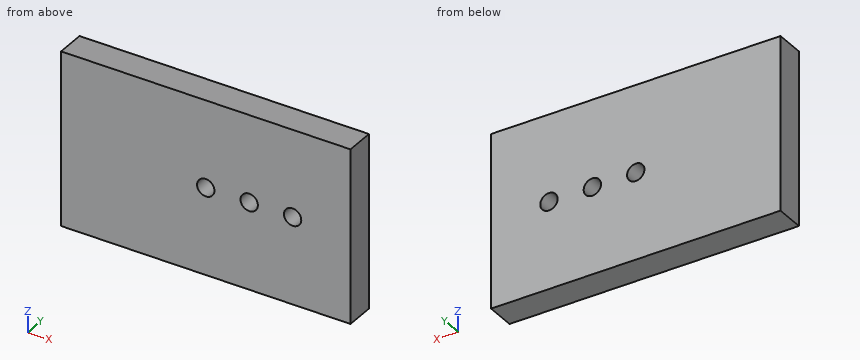
```python
from build123d import *

# Parameters (mm, degrees)
SKETCH_1_W             = 100
SKETCH_1_H             = 60
EXTRUDE_1_DEPTH        = 10
SKETCH_2_R             = 3
CUT_EXTRUDE_1_DEPTH    = 20
PATTERN_LINEAR_1_COUNT = 3
PATTERN_LINEAR_1_PITCH = 15


with BuildPart() as part:
    # 草图1 → 凸台-拉伸1 (new body)
    with BuildSketch(Plane(origin=(0, 0, 0), x_dir=(1, 0, 0), z_dir=(0, 1, 0))):
        Rectangle(SKETCH_1_W, SKETCH_1_H)
    extrude(amount=EXTRUDE_1_DEPTH)

    # 草图2 → 切除-拉伸1 (cut)
    with BuildSketch(Plane(origin=(0, 0, 0), x_dir=(1, 0, 0), z_dir=(0, 1, 0))):
        with Locations(Location((30, 0, 0), (0, 0, 90))):
            Circle(SKETCH_2_R)
    cut_extrude_1 = extrude(amount=CUT_EXTRUDE_1_DEPTH, mode=Mode.SUBTRACT)

    # 阵列(线性)1: 切除-拉伸1 ×3
    with Locations(*[(-i * PATTERN_LINEAR_1_PITCH, 0, 0) for i in range(1, PATTERN_LINEAR_1_COUNT)]):
        add(cut_extrude_1, mode=Mode.SUBTRACT)


solid = part.part
```
Part model, mm, in its own coordinate system. Give positions to 0.01 mm unless a question says otherwise; leave off trailing zeros. Order: outer loops, then holes, each group sorted by start corner. A loop starts at its lowest first (then second) coordinate and runs counter-clockwise, first axis right, second up. Notation, with made-up numbers: M 32,45.25 L 67,45.25 A29 ccw 67,78.25 Z; hole C 75,14.25 d11. An arc over 180 degrees is marked long. Use a Markdown table: item, result. Add a question column.
(1) Probe line 1 along X through (y, z) = (3, 0); line 2 along Z through (x, y) = (15, 7.5); line 3 along Z through (x, y) = (1.5, 2). List the from-to ranges inside material, lowest first. Write a range as [from, to].
(2) Saw through at B-B, the plane z = 0. Give the cut face in (x, y).
(3) Saw through at A-A, the plane x = 0. Give the cut face in (y, z), and give its area (3 significant figures).
(4) Drop a flat-ended pin along its axis: P1, Ø5.5, axis at x = 30, z = 0, coming from the -Y side. Give the stop position or say it passes through.
(5) Saw through at C-C, the plane x = 28. Give the cut face in (y, z), and give its area (3 significant figures).
Answer key:
| question | item | result |
|---|---|---|
| 1 | line 1 | [-50, -3], [3, 12], [18, 27], [33, 50] |
| 1 | line 2 | [-30, -3], [3, 30] |
| 1 | line 3 | [-30, -2.6], [2.6, 30] |
| 2 | outline | M -50,0 L -3,0 L -3,10 L -50,10 Z; M 3,0 L 12,0 L 12,10 L 3,10 Z; M 18,0 L 27,0 L 27,10 L 18,10 Z; M 33,0 L 50,0 L 50,10 L 33,10 Z |
| 3 | outline | M 0,-30 L 10,-30 L 10,-3 L 0,-3 Z; M 0,3 L 10,3 L 10,30 L 0,30 Z |
| 3 | area | 540 mm^2 |
| 4 | P1 | through |
| 5 | outline | M 0,-30 L 10,-30 L 10,-2.24 L 0,-2.24 Z; M 0,2.24 L 10,2.24 L 10,30 L 0,30 Z |
| 5 | area | 555 mm^2 |
